Part model, mm, in its own coordinate system. Face numbers are marked on the shaded views. A direction names the side the tool comes from. Give positions to 0.01 mm unless a question says otherwise; leave off trailing zeros. Order: outer loops, then holes, each group sorted by start corner. A loop starts at its lowest first (then second) coordinate and runs counter-clockwise, first axis right, second up. Notation, with made-up numbers: (52, 15) - (86, 15) arc R24 ccw to (86, 49) - close; hole circle Ø11 at (-22.75, 80). An arc over 180 degrees is marked (long way). One line per item, written item: value.
```python
from build123d import *

# Parameters (mm, degrees)
EXTRUDE_1_DEPTH     = 61.6
SHELL_1_T           = -2
FILLET_2_R          = 3
CUT_EXTRUDE_1_REACH = 88.192
SKETCH_3_W          = 4.6
SKETCH_3_H          = 7.4
SKETCH_4_W          = 4.6
SKETCH_4_H          = 7.4
EXTRUDE_2_DEPTH     = 1.7
SKETCH_5_W          = 2.95
SKETCH_5_H          = 7.9
SKETCH_5_W_2        = 25.755
SKETCH_5_H_2        = 2
EXTRUDE_3_DEPTH     = 1
EXTRUDE_4_DEPTH     = 7.897587
CUT_EXTRUDE_START   = -61.6
CUT_EXTRUDE_3_DEPTH = 61.6
CUT_EXTRUDE_START_2 = -54.8
CUT_EXTRUDE_4_DEPTH = 54.8
CUT_EXTRUDE_5_DEPTH = 3.5
CUT_EXTRUDE_6_DEPTH = 3.5


with BuildPart() as part:
    # ｽｹｯﾁ2 → ﾎﾞｽ - 押し出し1 (new body)
    with BuildSketch(Plane(origin=(0, 0, 0), x_dir=(0, 0, -1), z_dir=(1, 0, 0))):
        with BuildLine():
            Line((0, 0), (15.13, 0))
            ThreePointArc((15.13, 0), (22.201067812, 2.928932188), (25.13, 10))
            Line((25.13, 10), (25.13, 44.8))
            ThreePointArc((25.13, 44.8), (22.201067812, 51.871067812), (15.13, 54.8))
            Line((15.13, 54.8), (0, 54.8))
            Line((0, 54.8), (0, 0))
        make_face()
    extrude(amount=EXTRUDE_1_DEPTH)

    # ｼｪﾙ1
    shell_1_openings = [part.faces().sort_by_distance(p)[0] for p in [
        (30.8, 27.4, 0),
    ]]
    offset(amount=SHELL_1_T, openings=shell_1_openings, kind=Kind.INTERSECTION)

    # ﾌｨﾚｯﾄ2
    fillet_2_edges = [part.edges().sort_by_distance(p)[0] for p in [
        (61.6, 2.928932188, -22.201067812),
        (61.6, 27.4, -25.13),
        (61.6, 51.871067812, -22.201067812),
        (61.6, 54.8, -7.565),
        (0, 54.8, -7.565),
        (0, 51.871067812, -22.201067812),
        (0, 27.4, -25.13),
        (61.6, 0, -7.565),
        (0, 2.928932188, -22.201067812),
        (0, 0, -7.565),
    ]]
    fillet(fillet_2_edges, radius=FILLET_2_R)

    # ｽｹｯﾁ3 → ｶｯﾄ - 押し出し1 (cut, up to next)
    with BuildSketch(Plane(origin=(0, 0, -25.13), x_dir=(-1, 0, 0), z_dir=(0, 0, -1)), mode=Mode.PRIVATE) as cut_extrude_1_sk1:
        with Locations((-37.2975, 27.4)):
            Rectangle(SKETCH_3_W, SKETCH_3_H)
    cut_extrude_1_tool1 = extrude(cut_extrude_1_sk1.sketch, amount=-CUT_EXTRUDE_1_REACH, mode=Mode.PRIVATE) & part.part
    # ｽｹｯﾁ3 → ｶｯﾄ - 押し出し1 (cut, up to next)
    with BuildSketch(Plane(origin=(0, 0, -25.13), x_dir=(-1, 0, 0), z_dir=(0, 0, -1)), mode=Mode.PRIVATE) as cut_extrude_1_sk2:
        with Locations((-24.3025, 27.4)):
            Rectangle(SKETCH_3_W, SKETCH_3_H)
    cut_extrude_1_tool2 = extrude(cut_extrude_1_sk2.sketch, amount=-CUT_EXTRUDE_1_REACH, mode=Mode.PRIVATE) & part.part
    add(cut_extrude_1_tool1.solids().sort_by_distance((37.2975, 27.4, -25.13))[0], mode=Mode.SUBTRACT)
    add(cut_extrude_1_tool2.solids().sort_by_distance((24.3025, 27.4, -25.13))[0], mode=Mode.SUBTRACT)

    # ｽｹｯﾁ4 → ﾎﾞｽ - 押し出し2 (add)
    with BuildSketch(Plane.XY.offset(-23.13)):
        Polygon((17.9225, 15.575), (30.6725, 15.575), (43.6775, 15.575), (43.6775, 39.225), (30.6725, 39.225), (17.9225, 39.225), align=None)
        with Locations((24.3025, 27.4)):
            Rectangle(SKETCH_4_W, SKETCH_4_H, mode=Mode.SUBTRACT)
        with Locations((37.2975, 27.4)):
            Rectangle(SKETCH_4_W, SKETCH_4_H, mode=Mode.SUBTRACT)
    extrude(amount=EXTRUDE_2_DEPTH)

    # ｽｹｯﾁ5 → ﾎﾞｽ - 押し出し3 (add)
    with BuildSketch(Plane.XY.offset(-21.43)):
        with Locations((19.3975, 27.4)):
            Rectangle(SKETCH_5_W, SKETCH_5_H)
        with Locations((42.2025, 27.4)):
            Rectangle(SKETCH_5_W, SKETCH_5_H)
        with Locations((30.8, 38.225)):
            Rectangle(SKETCH_5_W_2, SKETCH_5_H_2)
        with Locations((30.8, 16.575)):
            Rectangle(SKETCH_5_W_2, SKETCH_5_H_2)
    extrude(amount=EXTRUDE_3_DEPTH)

    # ｽｹｯﾁ6 → ﾎﾞｽ - 押し出し4 (add)
    with BuildSketch(Plane(origin=(-6.518280687, 23.45241299, -44.223812227), x_dir=(1, 0, 0), z_dir=(0, 1, 0))):
        Polygon((34.190780687, -22.793812227), (40.445780687, -22.793812227), (40.445780687, -30.193812227), (42.170780687, -30.193812227), (42.170780687, -33.193812227), (32.465780687, -33.193812227), (32.465780687, -30.193812227), (34.190780687, -30.193812227), align=None)
    extrude(amount=EXTRUDE_4_DEPTH)

    # ｽｹｯﾁ8 → ｶｯﾄ - 押し出し3 (cut)
    with BuildSketch(Plane.ZY.offset(CUT_EXTRUDE_START)):
        with BuildLine():
            Line((0, 51.399152482), (0, 39.600847518))
            ThreePointArc((0, 39.600847518), (-3, 45.5), (0, 51.399152482))
        make_face()
        with BuildLine():
            Line((0, 15.199152482), (0, 3.400847518))
            ThreePointArc((0, 3.400847518), (-3, 9.3), (0, 15.199152482))
        make_face()
    extrude(amount=CUT_EXTRUDE_3_DEPTH, mode=Mode.SUBTRACT)

    # ｽｹｯﾁ9 → ｶｯﾄ - 押し出し4 (cut)
    with BuildSketch(Plane.XZ.offset(CUT_EXTRUDE_START_2)):
        with BuildLine():
            Line((56.299152482, 0), (44.500847518, 0))
            ThreePointArc((44.500847518, 0), (50.4, -3), (56.299152482, 0))
        make_face()
        with BuildLine():
            Line((17.099152482, 0), (5.300847518, 0))
            ThreePointArc((5.300847518, 0), (11.2, -3), (17.099152482, 0))
        make_face()
    extrude(amount=CUT_EXTRUDE_4_DEPTH, mode=Mode.SUBTRACT)

    # ｽｹｯﾁ11 → ｶｯﾄ - 押し出し5 (cut, symmetric)
    with BuildSketch(Plane(origin=(0, 27.4, 0), x_dir=(-1, 0, 0), z_dir=(0, -1, 0))):
        Polygon((-59.6, 1.176601917), (-59.6, 2.476687437), (-60.288664164, 1.788023273), (-60.288664164, 1.176601917), align=None)
        Polygon((-1.311335836, 1.176601917), (-2, 1.176601917), (-2, 2.476687437), (-1.311335836, 1.788023273), align=None)
    extrude(amount=CUT_EXTRUDE_5_DEPTH, both=True, mode=Mode.SUBTRACT)

    # ｽｹｯﾁ12 → ｶｯﾄ - 押し出し6 (cut, symmetric)
    with BuildSketch(Plane(origin=(30.8, 0, 0), x_dir=(0, 0, -1), z_dir=(1, 0, 0))):
        Polygon((2.501421356, 2), (1.201335836, 2), (1.201335836, 1.311335836), (1.812757192, 1.311335836), align=None)
        Polygon((1.812757192, 53.488664164), (2.501421356, 52.8), (1.201335836, 52.8), (1.201335836, 53.488664164), align=None)
    extrude(amount=CUT_EXTRUDE_6_DEPTH, both=True, mode=Mode.SUBTRACT)


solid = part.part
```
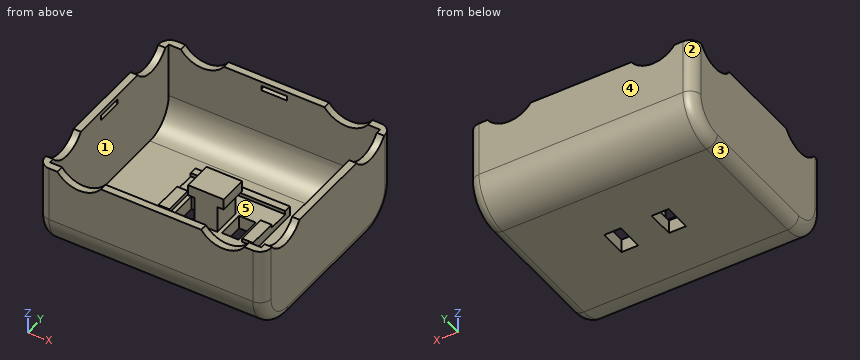
1) Slice it at A-A on z = -8.5. Write the cut outline in (x, y), then the cut area to 3 significant figures.
Answer:
outline: (0, 3) arc R3 ccw to (3, 0) - (58.6, 0) arc R3 ccw to (61.6, 3) - (61.6, 51.8) arc R3 ccw to (58.6, 54.8) - (3, 54.8) arc R3 ccw to (0, 51.8) - close; hole (2, 2) - (59.6, 2) - (59.6, 52.8) - (2, 52.8) - close
area: 442 mm2
2) Slice it at B-B on y = 33. Write the cut outline in (x, z).
Answer:
outline: (0, -22.13) arc R3 ccw to (3, -25.13) - (58.6, -25.13) arc R3 ccw to (61.6, -22.13) - (61.6, 0) - (59.6, 0) - (59.6, -23.13) - (43.68, -23.13) - (43.68, -21.43) - (17.92, -21.43) - (17.92, -23.13) - (2, -23.13) - (2, 0) - (0, 0) - close
3) Drop flat-ended pins along their axis: P1, Ø0.6, axis at x = 31, y = 17, coming from the +Z side; P2, Ø0.6, axis at y = 53.5, z = -2, coming from the +X side; P3, Ø1.8, axis at x = 37, z = -24, coming from the +Y side. Give the stop position or say it passes through.
Answer:
P1: stops at z = -20.43
P2: stops at x = 61.25
P3: stops at y = 50.84
4) Which spindle directions (+Z, -Z, +X, -X, +Y, -Y) get a long thin tool onto all of the face, cutting with end or side? Do the marked faces 1 and 2. Say none if no direction does.
Answer:
face 1: +Z
face 2: +Z, -Z, -X, +Y
5) Slice it at C-C on x = 16. Write the cut outline in (y, z).
Answer:
outline: (0, -15.13) arc R10 ccw to (10, -25.13) - (44.8, -25.13) arc R10 ccw to (54.8, -15.13) - (54.8, -1.2) - (52.8, -1.2) - (52.8, -15.13) arc R8 cw to (44.8, -23.13) - (10, -23.13) arc R8 cw to (2, -15.13) - (2, -1.2) - (0, -1.2) - close
6) Wall check: line 1 along X through (y, z) = (29.5, -15.75); line 2 along X through (y, z) = (39, -22); line 3 along X through (y, z) = (50.5, -10.75). Give the ranges that are in metal, low to high. Write a range as [from, to].
Answer:
line 1: x = [0, 2], [27.67, 33.93], [59.6, 61.6]
line 2: x = [0, 2], [17.92, 43.68], [59.6, 61.6]
line 3: x = [0, 2], [59.6, 61.6]
7) Two-plate mould, pull along X, no slides. Class the marked faces 3, 4 and 5: pulls with the +X half, pulls with the -X half, needs draft (parallel to the pull), parting line crosses it, or undercut.
Answer:
face 3: pulls with the -X half
face 4: needs draft
face 5: undercut
